from build123d import *

# Parameters (mm, degrees)
F0_W     = 5
F0_H     = 4
F1_DEPTH = 1
F2_W     = 1
F2_H     = 5
F3_DEPTH = 5
F4_R     = 4.99999
F2_H_2   = 14
F5_DEPTH = 5


# Not quite as in the source:
# - a fillet or chamfer is up to 0.001 mm smaller than in the source, because OpenCascade refuses the exact size


with BuildPart() as f1:
    # F0 (on Top) → F1 (new body)
    with BuildSketch(Plane.XY):
        Polygon((-4.5, -7), (-0.5, -7), (-0.5, -2), (-0.5, 2), (-0.5, 7), (-4.5, 7), align=None)
        with Locations((2, 0)):
            Rectangle(F0_W, F0_H)
    extrude(amount=F1_DEPTH)

    # F2 (on face) → F3 (join)
    with BuildSketch(Plane.XY.offset(1)):
        Polygon((-0.5, -2), (4.5, -2), (4.5, -1), (-1.5, -1), (-1.5, -2), align=None)
        with Locations((-1, -4.5)):
            Rectangle(F2_W, F2_H)
        Polygon((-1.5, 1), (4.5, 1), (4.5, 2), (-0.5, 2), (-1.5, 2), align=None)
        with Locations((-1, 4.5)):
            Rectangle(F2_W, F2_H)
    extrude(amount=F3_DEPTH)

    # F4 (radius 5 in the source; OpenCascade refuses exactly that, so slightly less here)
    f4_edges = [f1.edges().sort_by_distance(p)[0] for p in [
        (-0.5, -2, 3),
        (-1.5, 1, 3.5),
        (-1.5, -1, 3.5),
        (-0.5, 2, 3),
    ]]
    fillet(f4_edges, radius=F4_R)

    # F2 (on face) → F5 (join)
    with BuildSketch(Plane.XY.offset(1)):
        with Locations((-4, 0)):
            Rectangle(F2_W, F2_H_2)
    extrude(amount=F5_DEPTH)


solid = f1.part
Work out the finished part from the listing and answer in its coordinate system (mm). A direction names the side the tool comes from. Give positions to 0.01 mm unless a question says otherwise; leave off trailing zeros. Loops run counter-clockwise (first coordinate to the right, second up) from the corner with the lowest first, then second, coordinate; pieces in that order, holes last. Notation, with made-up numbers: M 40,28 L 51,28 A5 cw 51,35 Z; hole C 62,49.5 d7. An arc over 180 degrees is marked long. Use CSV: the item, a comma, the result in double quotes.
1) Find section B-B on y = 3.5. Write down the section's boundary in (x, z), plus the area to 3 significant figures.
Answer:
outline,"M -4.5,0 L 0.93,0 L 0.93,6 L -0.83,6 L -0.83,1 L -3.5,1 L -3.5,6 L -4.5,6 Z"
area,"19.2 mm^2"
2) Find section A-A on z = 2.3. Give the number of separate pieces and of enclosed holes in the cut face, plus the area to 3 significant figures.
Answer:
separate pieces,"3"
enclosed holes,"0"
area,"36.0 mm^2"
3) Given P1, Ø2, axis at x = 1, z = 3, coming from the -Y side; P2, Ø0.5, axis at x = 4, z = 3, coming from the -Y side, each flat-ended and moving along its own axis, determine where each tip first touches the part or whether it passes through.
Answer:
P1,"y = -4.82"
P2,"y = -2.06"
4) Find section D-D on x = -2.5. Write down the section's boundary in (y, z), plus the area to 3 significant figures.
Answer:
outline,"M -7,0 L 7,0 L 7,1 L -7,1 Z"
area,"14.0 mm^2"
5) Determine the mould class of faces 1 (the flat face through (4, -1, 3)), 2 (the flat face through (0.6, 3.6, 6)), 3 (the flat face through (-1, 0, 0)) for opening direction Z: released by +Z, released by -Z, zero draft, split by the parting line, or undercut.
Answer:
face 1,"zero draft"
face 2,"released by +Z"
face 3,"released by -Z"
6) Which of the six approach directions +Z, -Z, +X, -X, +Y, -Y give full straight-line access (tool end or side, diameter ignored) to faces 4 (the flat face through (4, 1, 3)), 5 (the cylindrical face through (-0.07, 2.5, 3.54)), 6 (the flat face through (-1.5, -6.5, 3.5)), 7 (the cylindrical face through (0.93, -3.5, 2.96))?
Answer:
face 4,"+Z, +X"
face 5,"+Z"
face 6,"+Z, +Y, -Y"
face 7,"+Z, -Z, +X, -Y"
7) Find section C-C on x = 2.5. Write down the section's boundary in (y, z), plus the area to 3 significant figures.
Answer:
outline,"M -2.42,0 L 2.42,0 L 2.42,6 L 1.1,6 L 1.1,1 L -1.1,1 L -1.1,6 L -2.42,6 Z"
area,"18.0 mm^2"
8) Consider L1, parallel to Z at x = -2, y = -0.75; L2, parallel to X at y = 2.5, z = 1.75; L3, parallel to X at y = 0.75, z = 1.4. Determine where each line is inside the solid, lowest interval first.
Answer:
L1,"0 to 1"
L2,"-4.5 to -3.5, -0.07 to 2.32"
L3,"-4.5 to -3.5"
